Geometry check sheet. Reference: drawing and pictorial views, mm from the part's lowest x, y, z. Round coordinates to 2 decimals unless told otherwise and drop trailing zeros. Write each loop counter-clockwise with the first axis right and the second up, starting at its lowest first coordinate (ties: lowest second). Pieces come first, ordered by that corner, then holes. Notation, with made-up numbers: (85.25, -11) -> (125.25, -11) arc R21 ccw to (125.25, 4) -> close; hole circle Ø9 at (-0.5, 28.25). An arc over 180 degrees is marked (long way). Answer as a JSON object with one key per item and string values. Group by question number.
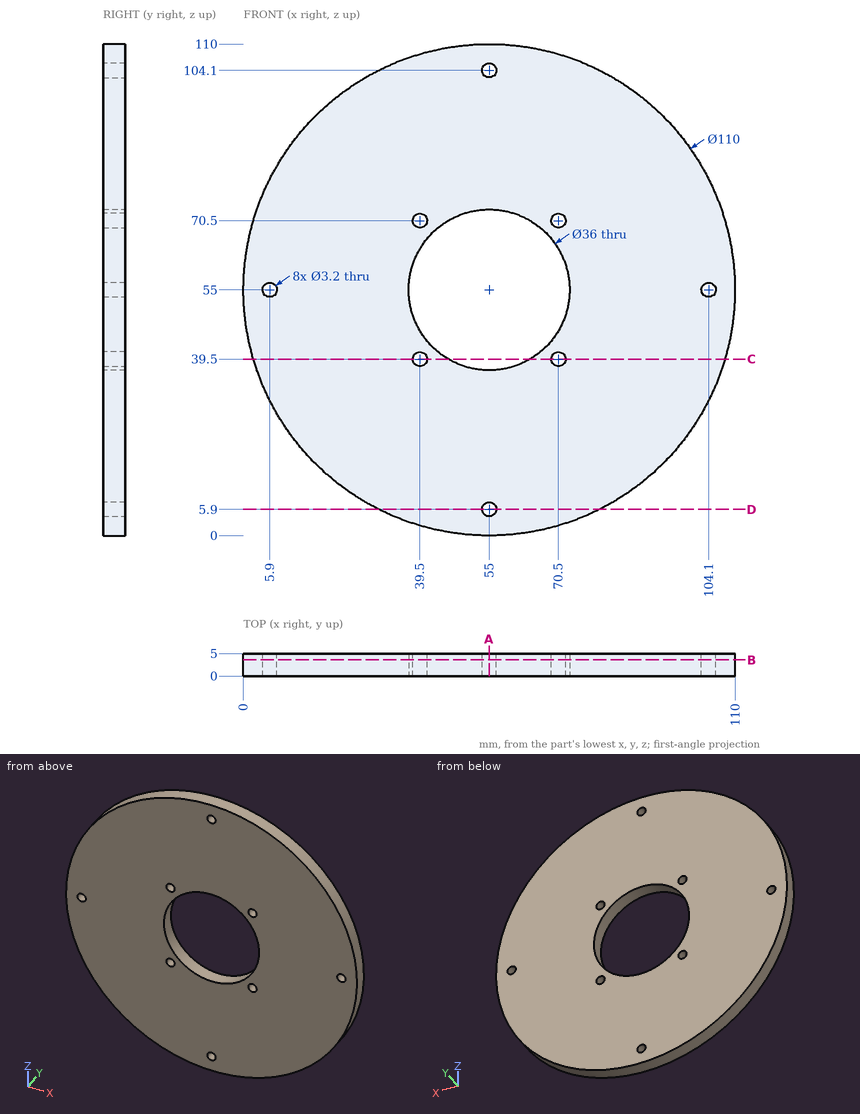
(1) Go/stop test with flat-tipped pins: pin 1 Ø2.5 at (x, z) = (70.5, 70.5) entering from +Y; pin 2 Ø1 at (y, z) = (2.5, 51) entering from -X; pin 3 Ø1.5 at (x, y) = (80.5, 3) entering from +Z; pin 4 Ø3 at (x, y) = (87.5, 3.5) entering from -Z. Record where each tip stops, or that it passes through.
(2) Scan lines: line 1 along X through (y, z) = (2.05, 55); line 2 along Z through (x, y) = (70.5, 1.55). Record each from-to range of solid material in increasing order.
(3) Section check A-A on x = 55. Record the cut outline in (y, z).
(4) Section check B-B on y = 3.6. State how many separate pieces and enclosed holes the cut face has, then the cut area to 3 significant figures.
(5) Section check C-C on z = 39.5. Record the cut outline in (x, y).
(6) Section check D-D on z = 5.9. Record the cut outline in (x, y).
Data:
{
 "1": {"pin 1": "passes through", "pin 2": "stops at x = 0.11", "pin 3": "stops at z = 104.12", "pin 4": "stops at z = 9.57"},
 "2": {"line 1": "x = 0 to 4.3, 7.5 to 37, 73 to 102.5, 105.7 to 110", "line 2": "z = 2.23 to 37.9, 41.1 to 45.85, 64.15 to 68.9, 72.1 to 107.77"},
 "3": {"outline": "(0, 0) -> (5, 0) -> (5, 4.3) -> (0, 4.3) -> close; (0, 7.5) -> (5, 7.5) -> (5, 37) -> (0, 37) -> close; (0, 73) -> (5, 73) -> (5, 102.5) -> (0, 102.5) -> close; (0, 105.7) -> (5, 105.7) -> (5, 110) -> (0, 110) -> close"},
 "4": {"separate pieces": "1", "enclosed holes": "9", "area": "8,420 mm²"},
 "5": {"outline": "(2.23, 0) -> (37.9, 0) -> (37.9, 5) -> (2.23, 5) -> close; (41.1, 0) -> (45.85, 0) -> (45.85, 5) -> (41.1, 5) -> close; (64.15, 0) -> (68.9, 0) -> (68.9, 5) -> (64.15, 5) -> close; (72.1, 0) -> (107.77, 0) -> (107.77, 5) -> (72.1, 5) -> close"},
 "6": {"outline": "(30.22, 0) -> (53.4, 0) -> (53.4, 5) -> (30.22, 5) -> close; (56.6, 0) -> (79.78, 0) -> (79.78, 5) -> (56.6, 5) -> close"}
}
